The listing builds one solid part. Answer for the finished solid, in the listing's coordinates (mm). A direction names the side the tool comes from. Coordinates: 2 decimals unless noted, no trailing zeros. Write each loop counter-clockwise with the first axis right and the second up, starting at its lowest first coordinate (ties: lowest second). Pieces come first, ordered by that corner, then holes.
from build123d import *

# Parameters (mm, degrees)
SKETCH1_W           = 330
SKETCH1_H           = 160
BOSS_EXTRUDE1_DEPTH = 260
SKETCH2_R           = 22
CUT_EXTRUDE1_DEPTH  = 25
SKETCH3_R           = 4.7625
CUT_EXTRUDE2_DEPTH  = 10


with BuildPart() as part:
    # Sketch1 → Boss-Extrude1 (new body)
    with BuildSketch(Plane(origin=(0, 0, 0), x_dir=(1, 0, 0), z_dir=(0, 1, 0))):
        Rectangle(SKETCH1_W, SKETCH1_H)
    extrude(amount=BOSS_EXTRUDE1_DEPTH)

    # Sketch2 → Cut-Extrude1 (cut)
    with BuildSketch(Plane(origin=(165, 0, 0), x_dir=(0, 0, -1), z_dir=(1, 0, 0))):
        with Locations((0, 150)):
            Circle(SKETCH2_R)
    extrude(amount=-CUT_EXTRUDE1_DEPTH, mode=Mode.SUBTRACT)

    # Sketch3 → Cut-Extrude2 (cut)
    with BuildSketch(Plane.XZ):
        with Locations(Location((82, 0, 0), (0, 0, 270))):
            Circle(SKETCH3_R)
        with Locations(Location((32, 0, 0), (0, 0, 270))):
            Circle(SKETCH3_R)
        with Locations(Location((-18, 0, 0), (0, 0, 270))):
            Circle(SKETCH3_R)
    extrude(amount=-CUT_EXTRUDE2_DEPTH, mode=Mode.SUBTRACT)


solid = part.part
1. Find the intervals of material crossed by L1, parallel to X at y = 3.75, z = 0; L2, parallel to X at y = 141.5, z = 18.5, in increasing order.
Results found:
L1: x = -165 to -22.76, -13.24 to 27.24, 36.76 to 77.24, 86.76 to 165
L2: x = -165 to 140
2. A tool of negligible diameter and unlimited length cuts with its end or side. For faces 4 (the cylindrical face through (86.72, 4.93, 0.62)), 5 (the flat face through (-2, 128, 80)), 6 (the cylindrical face through (152.675, 171.813, 2.864)), from which of +Z, -Z, +X, -X, +Y, -Y can it reach the whole face along a straight path? Write none if from no direction.
Results found:
face 4: -Y
face 5: +Z, +X, -X, +Y, -Y
face 6: +X
3. For a pull along X with two mould halves and no side action, classify faces 1 (the flat face through (165, 128, -17)), 2 (the flat face through (-165, 128, 1)), 3 (the flat face through (82, 10, 0)) as pulls with the +X half, pulls with the -X half, needs draft (parallel to the pull), parting line crosses it, or undercut.
Results found:
face 1: pulls with the +X half
face 2: pulls with the -X half
face 3: undercut
4. Section B-B on y = 140 is taken. Give the vertices of the cut face in (x, z).
Results found:
outline: (-165, -80) - (165, -80) - (165, -19.6) - (140, -19.6) - (140, 19.6) - (165, 19.6) - (165, 80) - (-165, 80) - close
5. Flat-ended cylindrical pins translate along their axes: P1, Ø13, axis at y = 159, z = 9.5, coming from the +X side; P2, Ø3, axis at x = 33.5, z = 0, coming from the -Y side. Find the tip coordinate at first contact, or state that the pin passes through.
Results found:
P1: stops at x = 140
P2: stops at y = 10
6. Section A-A on z = 0 is taken. Give the vertices of the cut face in (x, y).
Results found:
outline: (-165, 0) - (-22.76, 0) - (-22.76, 10) - (-13.24, 10) - (-13.24, 0) - (27.24, 0) - (27.24, 10) - (36.76, 10) - (36.76, 0) - (77.24, 0) - (77.24, 10) - (86.76, 10) - (86.76, 0) - (165, 0) - (165, 128) - (140, 128) - (140, 172) - (165, 172) - (165, 260) - (-165, 260) - close
